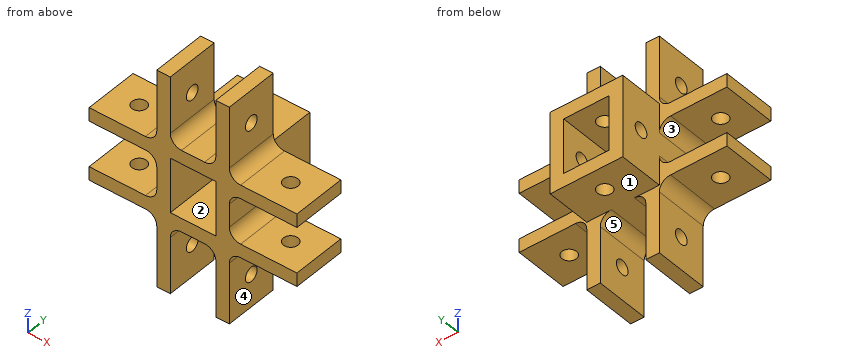
from build123d import *

# Parameters (mm, degrees)
ESQUISSE2_W               = 10.1
ESQUISSE2_H               = 12.1
BOSS_EXTRU_1_DEPTH        = 12
ENL_V_MAT_EXTRU_1_REACH   = 46.317
ESQUISSE3_R               = 1.6
SYM_TRIE6_COPY_1_REACH    = 46.317
SYM_TRIE6_COPY_1_SKETCH_R = 1.6
ESQUISSE4_W               = 16.1
ESQUISSE4_H               = 18.1
ESQUISSE4_W_2             = 10.1
ESQUISSE4_H_2             = 12.1
EXTRU_MINCE1_DEPTH        = 10
ESQUISSE5_R               = 1.6
ENL_V_MAT_EXTRU_2_DEPTH   = 49.674634051


with BuildPart() as part:
    # Esquisse2 → Boss.-Extru.1 (new body)
    with BuildSketch(Plane(origin=(0, 0, 0), x_dir=(1, 0, 0), z_dir=(0, 1, 0))):
        with BuildLine():
            Line((0, 11.55), (0, 24.05))
            Line((0, 24.05), (-3, 24.05))
            Line((-3, 24.05), (-3, 10.55))
            ThreePointArc((-3, 10.55), (-3.732233047, 8.782233047), (-5.5, 8.05))
            Line((-5.5, 8.05), (-18, 8.05))
            Line((-18, 8.05), (-18, 5.05))
            Line((-18, 5.05), (-5.5, 5.05))
            ThreePointArc((-5.5, 5.05), (-3.732233047, 4.317766953), (-3, 2.55))
            Line((-3, 2.55), (-3, -2.55))
            ThreePointArc((-3, -2.55), (-3.732233047, -4.317766953), (-5.5, -5.05))
            Line((-5.5, -5.05), (-18, -5.05))
            Line((-18, -5.05), (-18, -8.05))
            Line((-18, -8.05), (-5.5, -8.05))
            ThreePointArc((-5.5, -8.05), (-3.732233047, -8.782233047), (-3, -10.55))
            Line((-3, -10.55), (-3, -24.05))
            Line((-3, -24.05), (0, -24.05))
            Line((0, -24.05), (0, -11.55))
            ThreePointArc((0, -11.55), (0.732233047, -9.782233047), (2.5, -9.05))
            Line((2.5, -9.05), (7.6, -9.05))
            ThreePointArc((7.6, -9.05), (9.367766953, -9.782233047), (10.1, -11.55))
            Line((10.1, -11.55), (10.1, -24.05))
            Line((10.1, -24.05), (13.1, -24.05))
            Line((13.1, -24.05), (13.1, -10.55))
            ThreePointArc((13.1, -10.55), (13.832233047, -8.782233047), (15.6, -8.05))
            Line((15.6, -8.05), (28.1, -8.05))
            Line((28.1, -8.05), (28.1, -5.05))
            Line((28.1, -5.05), (15.6, -5.05))
            ThreePointArc((15.6, -5.05), (13.832233047, -4.317766953), (13.1, -2.55))
            Line((13.1, -2.55), (13.1, 2.55))
            ThreePointArc((13.1, 2.55), (13.832233047, 4.317766953), (15.6, 5.05))
            Line((15.6, 5.05), (28.1, 5.05))
            Line((28.1, 5.05), (28.1, 8.05))
            Line((28.1, 8.05), (15.6, 8.05))
            ThreePointArc((15.6, 8.05), (13.832233047, 8.782233047), (13.1, 10.55))
            Line((13.1, 10.55), (13.1, 24.05))
            Line((13.1, 24.05), (10.1, 24.05))
            Line((10.1, 24.05), (10.1, 11.55))
            ThreePointArc((10.1, 11.55), (9.367766953, 9.782233047), (7.6, 9.05))
            Line((7.6, 9.05), (2.5, 9.05))
            ThreePointArc((2.5, 9.05), (0.732233047, 9.782233047), (0, 11.55))
        make_face()
        with Locations((5.05, 0)):
            Rectangle(ESQUISSE2_W, ESQUISSE2_H, mode=Mode.SUBTRACT)
    extrude(amount=BOSS_EXTRU_1_DEPTH)

    # Enlèv. mat.-Extru.1: up to this face of the body (flat: up to its plane)
    enl_v_mat_extru_1_end = Plane(part.part.faces().sort_by_distance((-11.75, 6, -8.05))[0])
    # Esquisse3 → Enlèv. mat.-Extru.1 (cut, up to the picked face)
    with BuildSketch(Plane.XY.offset(8.05), mode=Mode.PRIVATE) as enl_v_mat_extru_1_sk1:
        with Locations((-11.75, 6)):
            Circle(ESQUISSE3_R)
    enl_v_mat_extru_1_tool1 = split(extrude(enl_v_mat_extru_1_sk1.sketch, amount=-ENL_V_MAT_EXTRU_1_REACH, mode=Mode.PRIVATE), bisect_by=enl_v_mat_extru_1_end, keep=Keep.BOTH, mode=Mode.PRIVATE)
    enl_v_mat_extru_1 = enl_v_mat_extru_1_tool1.solids().sort_by(Axis((-11.75, 6, 8.05), (0, 0, -1)))[0]
    add(enl_v_mat_extru_1, mode=Mode.SUBTRACT)

    # Symétrie1: Enlèv. mat.-Extru.1 across plane
    add(enl_v_mat_extru_1.mirror(Plane(origin=(5.05, 0, 0), x_dir=(0, 0, 1), z_dir=(1, 0, 0))), mode=Mode.SUBTRACT)

    # Symétrie6: Enlèv. mat.-Extru.1 across plane
    add(enl_v_mat_extru_1.mirror(Plane(origin=(2.525, 0, -2.525), x_dir=(0.7071067811865478, 0, 0.7071067811865472), z_dir=(-0.7071067811865475, 0, 0.7071067811865477))), mode=Mode.SUBTRACT)

    # Symétrie6 copy 1: up to this face of the body (flat: up to its plane)
    sym_trie6_copy_1_end = Plane(part.part.faces().sort_by_distance((-3, 6, 16.8))[0])
    # Symétrie6 copy 1 sketch → Symétrie6 copy 1 (cut, up to the picked face)
    with BuildSketch(Plane(origin=(13.1, 0, 5.05), x_dir=(0, 0, -1), z_dir=(1, 0, 0)), mode=Mode.PRIVATE) as sym_trie6_copy_1_sk1:
        with Locations((-11.75, 6)):
            Circle(SYM_TRIE6_COPY_1_SKETCH_R)
    sym_trie6_copy_1_tool1 = split(extrude(sym_trie6_copy_1_sk1.sketch, amount=-SYM_TRIE6_COPY_1_REACH, mode=Mode.PRIVATE), bisect_by=sym_trie6_copy_1_end, keep=Keep.BOTH, mode=Mode.PRIVATE)
    add(sym_trie6_copy_1_tool1.solids().sort_by(Axis((13.1, 6, 16.8), (-1, 0, 0)))[0], mode=Mode.SUBTRACT)

    # Esquisse4 → Extru.-Mince1 (add)
    with BuildSketch(Plane(origin=(0, 12, 0), x_dir=(1, 0, 0), z_dir=(0, 1, 0))):
        with Locations((5.05, 0)):
            Rectangle(ESQUISSE4_W, ESQUISSE4_H)
        with Locations((5.05, 0)):
            Rectangle(ESQUISSE4_W_2, ESQUISSE4_H_2, mode=Mode.SUBTRACT)
    extrude(amount=EXTRU_MINCE1_DEPTH)

    # Esquisse5 → Enlèv. mat.-Extru.2 (cut, through all)
    with BuildSketch(Plane(origin=(0, 0, -9.05), x_dir=(-1, 0, 0), z_dir=(0, 0, -1))):
        with Locations((-5.05, 17)):
            Circle(ESQUISSE5_R)
    enl_v_mat_extru_2 = extrude(amount=-ENL_V_MAT_EXTRU_2_DEPTH, mode=Mode.SUBTRACT)

    # Symétrie10: Enlèv. mat.-Extru.2 across plane
    add(enl_v_mat_extru_2.mirror(Plane(origin=(2.525, 0, -2.525), x_dir=(0.7071067811865478, 0, 0.7071067811865472), z_dir=(-0.7071067811865475, 0, 0.7071067811865477))), mode=Mode.SUBTRACT)


solid = part.part
Can you work these out from the model? Positions are in its coordinate system, mm. Face numbers are marked on the shaded views. A direction names the side the tool comes from. Coordinates: 2 decimals unless noted, no trailing zeros. Order: outer loops, then holes, each group sorted by start corner. A loop starts at its lowest first (then second) coordinate and runs counter-clockwise, first axis right, second up. Notation, with made-up numbers: (-31.75, 44.25) - (2.25, 44.25) arc R11 cw to (2.25, 52.25) - close; hole circle Ø7 at (46.5, -28.5). An arc over 180 degrees is marked (long way). Answer as a JSON object with one key per item and string values. Group by question number.
Q1. On a 3-axis mill with a long thin cutter (end or side, diameter ignored), from which of +Z, -Z, +X, -X, +Y, -Y can I reach the whole of each face in a straight line? I mean the marked faces 1, 2, 3, 4 and 5. Say none if no direction works.
Q2. I need wall thicknesses on line 1 (Y direction, x = -11.75, z = -6.85); line 2 (Z direction, x = 3.5, y = 4); line 3 (Z direction, x = 17.5, y = 3.5). Which ranges of each line are inside material? Lowest first, please. Write a range as from..to.
Q3. Imagine slicing it at A-A (z = 0). Please give me the cut outline in (x, y), and give its area (3 significant figures).
Q4. Will these pins go through, and if not, where does the flat tip stop? P1, Ø5, axis at x = 6.5, y = 16, coming from the +Z side; P2, Ø1.5, axis at y = 6.5, z = -11, coming from the -X side; P3, Ø3.5, axis at y = 8.5, z = 16, coming from the +X side.
Q5. Imagine slicing it at D-D (z = -20). Please give me the cut outline in (x, y).
Q6. Imagine slicing it at C-C (y = 17). Please give me the cut outline in (x, z).
Q7. Imagine slicing it at B-B (x = -8.5). Please give me the cut outline in (y, z), and give its area (3 significant figures).
Determined:
{
 "1": {"face 1": "-Z, +Y", "face 2": "+Y, -Y", "face 3": "-X, +Y, -Y", "face 4": "-Z, +X, +Y, -Y", "face 5": "-Z, +Y, -Y"},
 "2": {"line 1": "y = 0..4.4, 7.6..12", "line 2": "z = -9.05..-6.05, 6.05..9.05", "line 3": "z = -8.05..-5.05, 5.05..8.05"},
 "3": {"outline": "(-3, 0) - (0, 0) - (0, 15.4) - (-3, 15.4) - close; (-3, 18.6) - (0, 18.6) - (0, 22) - (-3, 22) - close; (10.1, 0) - (13.1, 0) - (13.1, 15.4) - (10.1, 15.4) - close; (10.1, 18.6) - (13.1, 18.6) - (13.1, 22) - (10.1, 22) - close", "area": "113 mm2"},
 "4": {"P1": "stops at z = 9.05", "P2": "stops at x = -3.02", "P3": "stops at x = 13.1"},
 "5": {"outline": "(-3, 0) - (0, 0) - (0, 12) - (-3, 12) - close; (10.1, 0) - (13.1, 0) - (13.1, 12) - (10.1, 12) - close"},
 "6": {"outline": "(-3, -9.05) - (3.45, -9.05) - (3.45, -6.05) - (0, -6.05) - (0, -1.6) - (-3, -1.6) - close; (-3, 1.6) - (0, 1.6) - (0, 6.05) - (3.45, 6.05) - (3.45, 9.05) - (-3, 9.05) - close; (6.65, -9.05) - (13.1, -9.05) - (13.1, -1.6) - (10.1, -1.6) - (10.1, -6.05) - (6.65, -6.05) - close; (6.65, 6.05) - (10.1, 6.05) - (10.1, 1.6) - (13.1, 1.6) - (13.1, 9.05) - (6.65, 9.05) - close"},
 "7": {"outline": "(0, -8.05) - (12, -8.05) - (12, -5.05) - (0, -5.05) - close; (0, 5.05) - (12, 5.05) - (12, 8.05) - (0, 8.05) - close", "area": "72.0 mm2"}
}
